Geometry check sheet. Reference: the model listing, model coordinates, mm. A direction names the side the tool comes from. Round coordinates to 2 decimals unless told otherwise and drop trailing zeros. Order: outer loops, then holes, each group sorted by start corner. A loop starts at its lowest first (then second) coordinate and runs counter-clockwise, first axis right, second up.
```python
from build123d import *

# Parameters (mm, degrees)
SKETCH1_R           = 11
BOSS_EXTRUDE2_DEPTH = 8
SKETCH3_R           = 3
SKETCH3_R_2         = 1.5
CUT_EXTRUDE2_DEPTH  = 12
CUT_EXTRUDE3_START  = -4
SKETCH4_R           = 11
SKETCH4_R_2         = 4.5
CUT_EXTRUDE3_DEPTH  = 4


with BuildPart() as part:
    # Sketch1 → Boss-Extrude2 (new body)
    with BuildSketch(Plane(origin=(0, 0, 0), x_dir=(1, 0, 0), z_dir=(0, 1, 0))):
        with Locations(Location((0, 0, 0), (0, 0, 270))):
            Circle(SKETCH1_R)
    extrude(amount=BOSS_EXTRUDE2_DEPTH)

    # Sketch3 → Cut-Extrude2 (cut)
    with BuildSketch(Plane(origin=(0, 8, 0), x_dir=(1, 0, 0), z_dir=(0, 1, 0))):
        with Locations(Location((0, 0, 0), (0, 0, 270))):
            Circle(SKETCH3_R)
        with Locations(Location((-7, 0, 0), (0, 0, 270))):
            Circle(SKETCH3_R_2)
        with Locations(Location((0, 7, 0), (0, 0, 270))):
            Circle(SKETCH3_R_2)
        with Locations(Location((7, 0, 0), (0, 0, 270))):
            Circle(SKETCH3_R_2)
        with Locations(Location((0, -7, 0), (0, 0, 270))):
            Circle(SKETCH3_R_2)
    extrude(amount=-CUT_EXTRUDE2_DEPTH, mode=Mode.SUBTRACT)

    # Sketch4 → Cut-Extrude3 (cut)
    with BuildSketch(Plane(origin=(0, 8, 0), x_dir=(1, 0, 0), z_dir=(0, 1, 0)).offset(CUT_EXTRUDE3_START)):
        with Locations(Location((0, 0, 0), (0, 0, 270))):
            Circle(SKETCH4_R)
        with Locations(Location((0, 0, 0), (0, 0, 270))):
            Circle(SKETCH4_R_2, mode=Mode.SUBTRACT)
    extrude(amount=CUT_EXTRUDE3_DEPTH, mode=Mode.SUBTRACT)


solid = part.part
```
(1) Sectioned sample at B-B, the plane x = 0.75. Record the cut outline in (y, z).
Returned:
outline: (0, -10.97) - (4, -10.97) - (4, -8.3) - (0, -8.3) - close; (0, -5.7) - (4, -5.7) - (4, -4.44) - (8, -4.44) - (8, -2.9) - (0, -2.9) - close; (0, 2.9) - (8, 2.9) - (8, 4.44) - (4, 4.44) - (4, 5.7) - (0, 5.7) - close; (0, 8.3) - (4, 8.3) - (4, 10.97) - (0, 10.97) - close
(2) Sectioned sample at A-A, the plane z = 0. Record the cut outline in (x, y), and give its area (3 significant figures).
Returned:
outline: (-11, 0) - (-8.5, 0) - (-8.5, 4) - (-11, 4) - close; (-5.5, 0) - (-3, 0) - (-3, 8) - (-4.5, 8) - (-4.5, 4) - (-5.5, 4) - close; (3, 0) - (5.5, 0) - (5.5, 4) - (4.5, 4) - (4.5, 8) - (3, 8) - close; (8.5, 0) - (11, 0) - (11, 4) - (8.5, 4) - close
area: 52.0 mm2
(3) Material ranges on line 1 (X direction, y = 0.75, z = 0); line 2 (Y direction, x = 4.5, z = 8.5); line 3 (X direction, y = 2.6, z = 7), recorded low to high.
Returned:
line 1: x = -11 to -8.5, -5.5 to -3, 3 to 5.5, 8.5 to 11
line 2: y = 0 to 4
line 3: x = -8.49 to -1.5, 1.5 to 8.49
(4) Draft check along Z on faces 3 (the flat face through (-3, 8, 1)), 4 (the cylindrical face through (0.9, 4.06, 2.86)), 5 (the cylindrical face through (-10.74, 1.97, -2.38)), 6 (the cylindrical face through (0.07, 2.03, -8.5)). Enter one of: released by +Z, released by -Z, zero draft, split by the parting line, or undercut.
Returned:
face 3: zero draft
face 4: undercut
face 5: split by the parting line
face 6: undercut
(5) Set-up check for faces 1 (the cylindrical face through (-8.464, 2.028, -0.325)), 2 (the cylindrical face through (1.352, 5.972, 4.292)): record each of +Z, -Z, +X, -X, +Y, -Y from which the full face is reachable in a straight line by a thin tool's end or side.
Returned:
face 1: +Y, -Y
face 2: +Y
(6) Depth check by flat-ended pin: P1, Ø4, axis at x = -5.5, z = -7, coming from the +Y side; P2, Ø2, axis at x = -2, y = 2, coming from the -Z side. Enter the tip coordinate at first touch or a pass-through.
Returned:
P1: stops at y = 4
P2: stops at z = -10.95
(7) Sectioned sample at D-D, the plane y = 3.5. Record the cut outline in (x, z), and give its area (3 significant figures).
Returned:
outline: circle Ø22 at (0, 0); hole circle Ø3 at (-7, 0); hole circle Ø6 at (0, 0); hole circle Ø3 at (0, -7); hole circle Ø3 at (0, 7); hole circle Ø3 at (7, 0)
area: 324 mm2
(8) Sectioned sample at C-C, the plane z = -7. Record the cut outline in (x, y).
Returned:
outline: (-8.49, 0) - (-1.5, 0) - (-1.5, 4) - (-8.49, 4) - close; (1.5, 0) - (8.49, 0) - (8.49, 4) - (1.5, 4) - close
